```python
from build123d import *

# Parameters (mm, degrees)
SKETCH1_W           = 50
SKETCH1_H           = 20
BOSS_EXTRUDE1_DEPTH = 0.5
SKETCH2_R           = 2
BOSS_EXTRUDE2_DEPTH = 25
SKETCH3_R           = 1
BOSS_EXTRUDE3_DEPTH = 20
BOSS_EXTRUDE4_START = -25
BOSS_EXTRUDE4_DEPTH = 50
SKETCH5_R           = 2
CUT_EXTRUDE1_DEPTH  = 29.761954037


# Read off the part's stored shape, not the designer's step: Boss-Extrude4
with BuildPart() as part:
    # Sketch1 → Boss-Extrude1 (new, symmetric)
    with BuildSketch(Plane(origin=(0, 0, 0), x_dir=(1, 0, 0), z_dir=(0, 1, 0))):
        Rectangle(SKETCH1_W, SKETCH1_H)
    extrude(amount=BOSS_EXTRUDE1_DEPTH, both=True)



with BuildPart() as body_2:
    # Sketch2 → Boss-Extrude2 (new body)
    with BuildSketch(Plane(origin=(25, 0, 0), x_dir=(0, 0, -1), z_dir=(1, 0, 0))):
        with Locations((12, 0)):
            Circle(SKETCH2_R)
    extrude(amount=-BOSS_EXTRUDE2_DEPTH)

    # Sketch3 → Boss-Extrude3 (add)
    with BuildSketch(Plane.ZY):
        with Locations(Location((-12, 0, 0), (0, 0, 180))):
            Circle(SKETCH3_R)
    extrude(amount=BOSS_EXTRUDE3_DEPTH)


with BuildPart() as part_1:
    add(part.part)

    add(body_2.part)  # Boss-Extrude4 merges body 2
    # Boss-Extrude4 outline → Boss-Extrude4 (add)
    with BuildSketch(Plane.YZ.offset(BOSS_EXTRUDE4_START)):
        with BuildLine():
            ThreePointArc((0, -10), (0.252008585, -10.015940607), (0.5, -10.063508327))
            Line((0.5, -10.063508327), (0.5, -10))
            Line((0.5, -10), (0, -10))
        make_face()
        with BuildLine():
            ThreePointArc((-0.5, -10.063508327), (-0.252008585, -10.015940607), (0, -10))
            Line((0, -10), (-0.5, -10))
            Line((-0.5, -10), (-0.5, -10.063508327))
        make_face()
    extrude(amount=BOSS_EXTRUDE4_DEPTH)

    # Sketch5 → Cut-Extrude1 (cut, through all)
    with BuildSketch(Plane(origin=(0, 0.5, 0), x_dir=(1, 0, 0), z_dir=(0, 1, 0))):
        with Locations(Location((9.5, 0, 0), (0, 0, 270))):
            Circle(SKETCH5_R)
        with Locations(Location((-9.5, 0, 0), (0, 0, 90))):
            Circle(SKETCH5_R)
    extrude(amount=-CUT_EXTRUDE1_DEPTH, mode=Mode.SUBTRACT)


solid = part_1.part
```
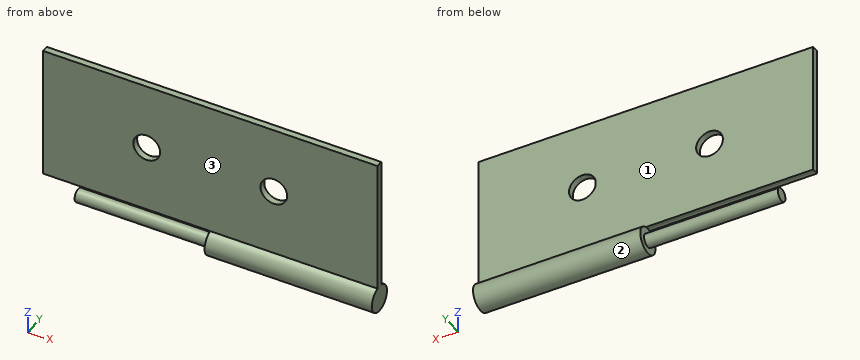
Here's how the part is built. I have some questions about the finished solid (model axes, mm). Face numbers are marked on the shaded views. A direction names the side the tool comes from. Give positions to 0.01 mm unless a question says otherwise; leave off trailing zeros. Loops run counter-clockwise (first coordinate to the right, second up) from the corner with the lowest first, then second, coordinate; pieces in that order, holes last. Notation, with made-up numbers: M 58.5,57 L 106.5,57 A30 cw 106.5,86 Z; hole C 50.25,41.5 d8. An arc over 180 degrees is marked long. Put each result on its own line as item: value. Start each with the question number.
(1) I want a section at A-A on x = 9.5. Please give me the cut outline in (y, z), then the cut area to 3 significant figures.
(2) Will these pins go through, and if not, where does the flat tip stop? pin 1 Ø1 at (x, z) = (-15, -8) entering from -Y; pin 2 Ø1.2 at (y, z) = (0.5, -12.5) entering from -X; pin 3 Ø5 at (x, z) = (9.5, 0) entering from +Y.
(3) I want a section at C-C on x = -9.5. Please give me the cut outline in (y, z).
(4) I want a section at B-B on z = 0. Please give me the cut outline in (x, y), then the cut area to 3 significant figures.
(5) I need wall thicknesses on line 1 along X through (y, z) = (0.05, 0); line 2 along Z through (x, y) = (-9.5, 0.3); line 3 along Y through (x, z) = (-19, 9). Which ranges of each line are inside material? Lowest first, please. Write a range as [from, to].
(6) For the marked faces 1, 2 and 3, which set-ups out of +Z, -Z, +X, -X, +Y, -Y let a thin tool reach every point of the face, with its end or its side?
(7) I want a section at D-D on z = -12. Please give me the cut outline in (x, y), then the cut area to 3 significant figures.
Answer block:
1. outline: M -0.5,-10.06 A2 ccw long 0.5,-10.06 L 0.5,-2 L -0.5,-2 Z; M -0.5,2 L 0.5,2 L 0.5,10 L -0.5,10 Z
1. area: 28.6 mm^2
2. pin 1: y = -0.5
2. pin 2: x = -20
2. pin 3: y = 0.5
3. outline: C 0,-12 d2; M -0.5,-10.06 A2 cw 0.5,-10.06 L 0.5,-2 L -0.5,-2 Z; M -0.5,2 L 0.5,2 L 0.5,10 L -0.5,10 Z
4. outline: M -25,-0.5 L -11.5,-0.5 L -11.5,0.5 L -25,0.5 Z; M -7.5,-0.5 L 7.5,-0.5 L 7.5,0.5 L -7.5,0.5 Z; M 11.5,-0.5 L 25,-0.5 L 25,0.5 L 11.5,0.5 Z
4. area: 42.0 mm^2
5. line 1: [-25, -11.5], [-7.5, 7.5], [11.5, 25]
5. line 2: [-12.95, -11.05], [-10.02, -2], [2, 10]
5. line 3: [-0.5, 0.5]
6. face 1: +Z, +X, -X, +Y
6. face 2: +X, -X
6. face 3: +Z, +X, -X, -Y
7. outline: M -20,-1 L 0,-1 L 0,-2 L 25,-2 L 25,2 L 0,2 L 0,1 L -20,1 Z
7. area: 140 mm^2
